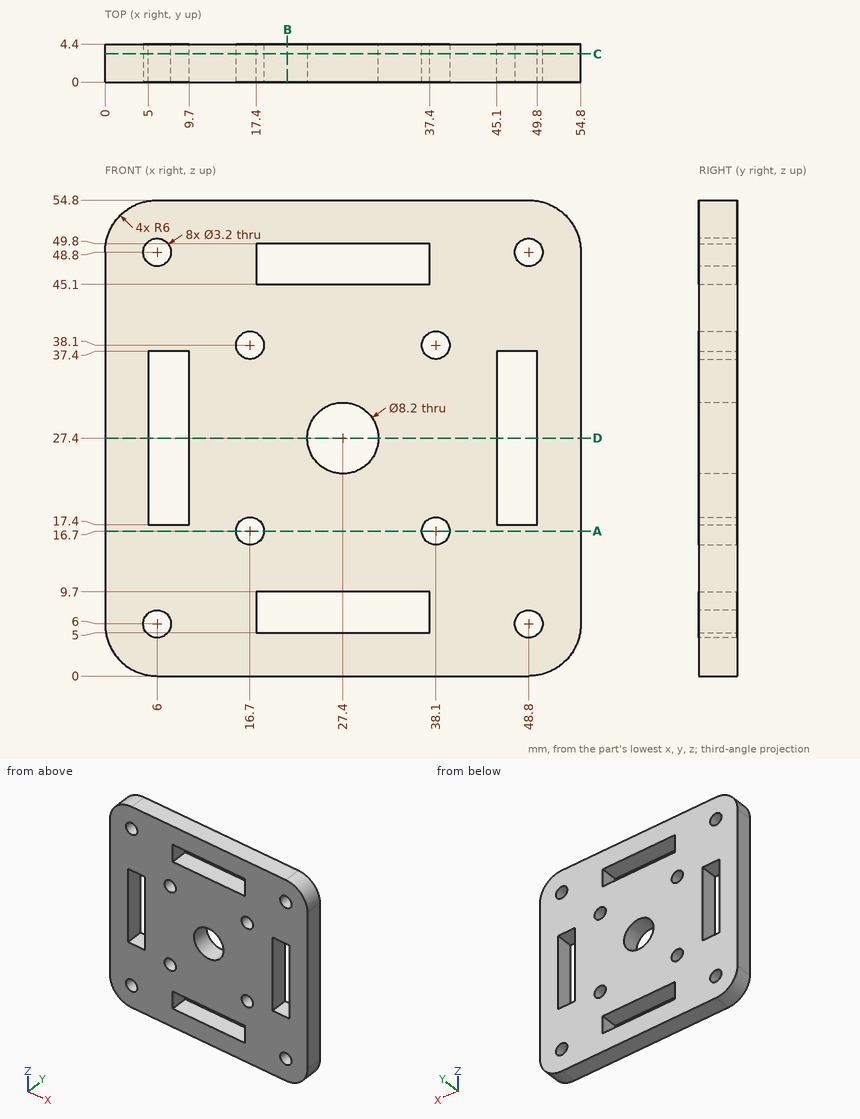
Geometry check sheet. Reference: drawing and pictorial views, mm from the part's lowest x, y, z. Coordinates: 2 decimals unless noted, no trailing zeros. Write each loop counter-clockwise with the first axis right and the second up, starting at its lowest first coordinate (ties: lowest second). Pieces come first, ordered by that corner, then holes. Notation, with made-up numbers: M 4.5,65 L 61.5,65 A7 cw 61.5,75 Z; hole C 72,18.5 d11. An arc over 180 degrees is marked long. Write item = value, one per line. Start each with the question number.
1. Sectioned sample at C-C (y = 3.25). State how many separate pieces and enclosed holes the cut face has, then the cut area to 3 significant figures.
2. Sectioned sample at B-B (x = 21). Record the cut outline in (y, z), then the cut area to 3 significant figures.
3. Sectioned sample at A-A (z = 16.7). Record the cut outline in (x, y), then the cut area to 3 significant figures.
4. Go/stop test with a flat-tipped pin: pin 1 (1.9 mm diameter, centred on x = 48.8, z = 48.8, fed in from -Y). Record where the tip stops, or that it passes through.
5. Thickness scan on probe 1 along X at (y, z) = (2.35, 16.7); probe 2 along Z at (x, y) = (48.8, 2.7). Record the ranges inside material, lowest first.
6. Sectioned sample at D-D (z = 27.4). Record the cut outline in (x, y), then the cut area to 3 significant figures.
The answers:
q1.separate_pieces = 1
q1.enclosed_holes = 13
q1.area = 2,480 mm²
q2.outline = M 0,0 L 4.4,0 L 4.4,5 L 0,5 Z; M 0,9.7 L 4.4,9.7 L 4.4,45.1 L 0,45.1 Z; M 0,49.8 L 4.4,49.8 L 4.4,54.8 L 0,54.8 Z
q2.area = 200 mm²
q3.outline = M 0,0 L 15.1,0 L 15.1,4.4 L 0,4.4 Z; M 18.3,0 L 36.5,0 L 36.5,4.4 L 18.3,4.4 Z; M 39.7,0 L 54.8,0 L 54.8,4.4 L 39.7,4.4 Z
q3.area = 213 mm²
q4.pin_1 = through
q5.probe_1 = 0 to 15.1, 18.3 to 36.5, 39.7 to 54.8
q5.probe_2 = 0 to 4.4, 7.6 to 17.4, 37.4 to 47.2, 50.4 to 54.8
q6.outline = M 0,0 L 5,0 L 5,4.4 L 0,4.4 Z; M 9.7,0 L 23.3,0 L 23.3,4.4 L 9.7,4.4 Z; M 31.5,0 L 45.1,0 L 45.1,4.4 L 31.5,4.4 Z; M 49.8,0 L 54.8,0 L 54.8,4.4 L 49.8,4.4 Z
q6.area = 164 mm²
